from build123d import *

# Parameters (mm, degrees)
F0_R     = 30.553649
F1_DEPTH = 8.128
F2_R     = 6.018054
F3_DEPTH = 28.448
F4_R     = 2.54


with BuildPart() as f1:
    # F0 (on Front) → F1 (new body, symmetric)
    with BuildSketch(Plane.XZ):
        with BuildLine():
            ThreePointArc((15.581804, -48.351291), (41.062122, -29.908898), (50.8, 0))
            ThreePointArc((50.8, 0), (41.062122, 29.908898), (15.581804, 48.351291))
            ThreePointArc((15.581804, 48.351291), (-50.8, 0), (15.581804, -48.351291))
        make_face()
        Circle(F0_R, mode=Mode.SUBTRACT)
        with BuildLine():
            ThreePointArc((15.581804, 48.351291), (41.062122, 29.908898), (50.8, 0))
            ThreePointArc((50.8, 0), (41.062122, -29.908898), (15.581804, -48.351291))
            Line((15.581804, -48.351291), (126.609508, -21.197307))
            ThreePointArc((126.609508, -21.197307), (99.603244, 0), (126.609508, 21.197307))
            Line((126.609508, 21.197307), (15.581804, 48.351291))
        make_face()
        with BuildLine():
            ThreePointArc((143.247345, 0), (138.591134, 13.473524), (126.609508, 21.197307))
            ThreePointArc((126.609508, 21.197307), (99.603244, 0), (126.609508, -21.197307))
            ThreePointArc((126.609508, -21.197307), (138.591134, -13.473524), (143.247345, 0))
        make_face()
    extrude(amount=F1_DEPTH, both=True)

    # F2 (on face) → F3 (join)
    with BuildSketch(Plane(origin=(12.037263, 0, 49.218178), x_dir=(0.971371, 0, -0.237568), z_dir=(0.237568, 0, 0.971371))):
        with Locations((62.131673, 0)):
            Circle(F2_R)
    extrude(amount=F3_DEPTH)

    # F4
    f4_edges = [f1.edges().sort_by_distance(p)[0] for p in [
        (73.302729, 0, 63.520958),
        (66.544404, 0, 35.887396),
    ]]
    fillet(f4_edges, radius=F4_R)


solid = f1.part
Here's how the part is built. I have some questions about the finished solid (model axes, mm). Coordinates: 2 decimals unless noted, no trailing zeros. Order: outer loops, then holes, each group sorted by start corner. A loop starts at its lowest first (then second) coordinate and runs counter-clockwise, first axis right, second up. Notation, with made-up numbers: (41, 38.25) -> (59, 38.25) arc R21 cw to (59, 67.25) -> close; hole circle Ø7 at (33.25, 84.25). An arc over 180 degrees is marked (long way). Answer in a Markdown table with one row per item.
(1) Please list where these lines run through material, in increasing order: probe 1 along Z at (x, y) = (0, -2.5); probe 2 along Z at (x, y) = (-20, -2.5); probe 3 along X at (y, z) = (0.75, 6).
Answer key:
| item | result |
|---|---|
| probe 1 | -50.8 to -30.55, 30.55 to 50.8 |
| probe 2 | -46.7 to -23.1, 23.1 to 46.7 |
| probe 3 | -50.44 to -29.96, 29.96 to 142.41 |
(2) Thinking about a two-plate mould opening in X: for faces 1 (the face through (70.318, -0.114, -34.964)), 2 (the face through (45, 8.128, 1)), 3 (the face through (16.43, 0.11, 25.76)), which applies, +X half, -X half, draft (parallel to the pull), parting line (faces both ways), or undercut?
Answer key:
| item | result |
|---|---|
| face 1 | +X half |
| face 2 | draft |
| face 3 | undercut |
(3) I want a section at A-A on x = 0. List the corners of the cut face in (y, z) for me, then the cut area to 3 significant figures.
Answer key:
| item | result |
|---|---|
| outline | (-8.13, -50.8) -> (8.13, -50.8) -> (8.13, -30.55) -> (-8.13, -30.55) -> close; (-8.13, 30.55) -> (8.13, 30.55) -> (8.13, 50.8) -> (-8.13, 50.8) -> close |
| area | 658 mm^2 |
(4) I want a section at C-C on x = 104.5. List the corners of the cut face in (y, z) for me, then the cut area to 3 significant figures.
Answer key:
| item | result |
|---|---|
| outline | (-8.13, -26.6) -> (8.13, -26.6) -> (8.13, 26.6) -> (-8.13, 26.6) -> close |
| area | 865 mm^2 |
(5) I want a section at B-B on z = 18.5. List the corners of the cut face in (x, y) for me, then the cut area to 3 significant figures.
Answer key:
| item | result |
|---|---|
| outline | (-47.31, -8.13) -> (-24.32, -8.13) -> (-24.32, 8.13) -> (-47.31, 8.13) -> close; (24.32, -8.13) -> (133, -8.13) -> (133, 8.13) -> (24.32, 8.13) -> close |
| area | 2,140 mm^2 |
(6) Will these pins go through, and if not, where does the flat tip stop? pin 1 Ø6 at (x, y) = (29, 6.5) entering from +Z; pin 2 Ø1.5 at (x, y) = (-28.5, -1) entering from +Z; pin 3 Ø1 at (y, z) = (1.5, -8.5) entering from -X.
Answer key:
| item | result |
|---|---|
| pin 1 | z = 45.8 |
| pin 2 | z = 42.55 |
| pin 3 | x = -50.17 |
